Job drawing, mm, ordinate dimensions from the low corner. One solid piece. A direction names the side the tool comes from. Give positions to 0.01 mm unless a question says otherwise; leave off trailing zeros. Order: outer loops, then holes, each group sorted by start corner. A loop starts at its lowest first (then second) coordinate and runs counter-clockwise, first axis right, second up. Notation, with made-up numbers: M 58,40.25 L 70,40.25 A19 ccw 70,53.25 Z; hole C -1.75,-13 d11. An arc over 180 degrees is marked long. Put each result on its own line as item: value. Start each with the question number.
1) Cut at C-C (z = 23.5). Write the cut outline in (x, y), and give its area (3 significant figures).
2) Cut at A-A (y = 73). Write the cut outline in (x, z), and give its area (3 significant figures).
3) Two-plate mould, pull along Z, no slides. Class the marked faces 1, 2 and 3: released by +Z, released by -Z, zero draft, split by the parting line, or undercut.
4) Cut at D-D (x = 21.5). Write the cut outline in (y, z).
5) Cut at B-B (z = 33.5). Write the cut outline in (x, y), and give its area (3 significant figures).
6) Drill centre lines: line 1 (X direction, y = 73, z = 36.75); line 2 (Y direction, x = 15, z = 25.25); line 3 (Z direction, x = 2.25, y = 83.5). Where is each one in solid material? Low to high. Write a range as [from, to].
7) Pin check, flat tips, straight feed: pin 1 (3 mm diameter, centred on x = 15, y = 5, fed in from +Z); pin 2 (1.2 mm diameter, centred on x = 1.5, z = 29, fed in from +Y); pin 3 (1 mm diameter, centred on x = 26, z = 16, fed in from -Y); pin 4 (3 mm diameter, centred on x = 6, z = 26.5, fed in from -Y). Stop position of each tip, or through.
8) Tool access for the marked faces 4, 5 and 6: list every direction of +Z, -Z, +X, -X, +Y, -Y with a clear straight run to the whole face (end or side of a thin tool).
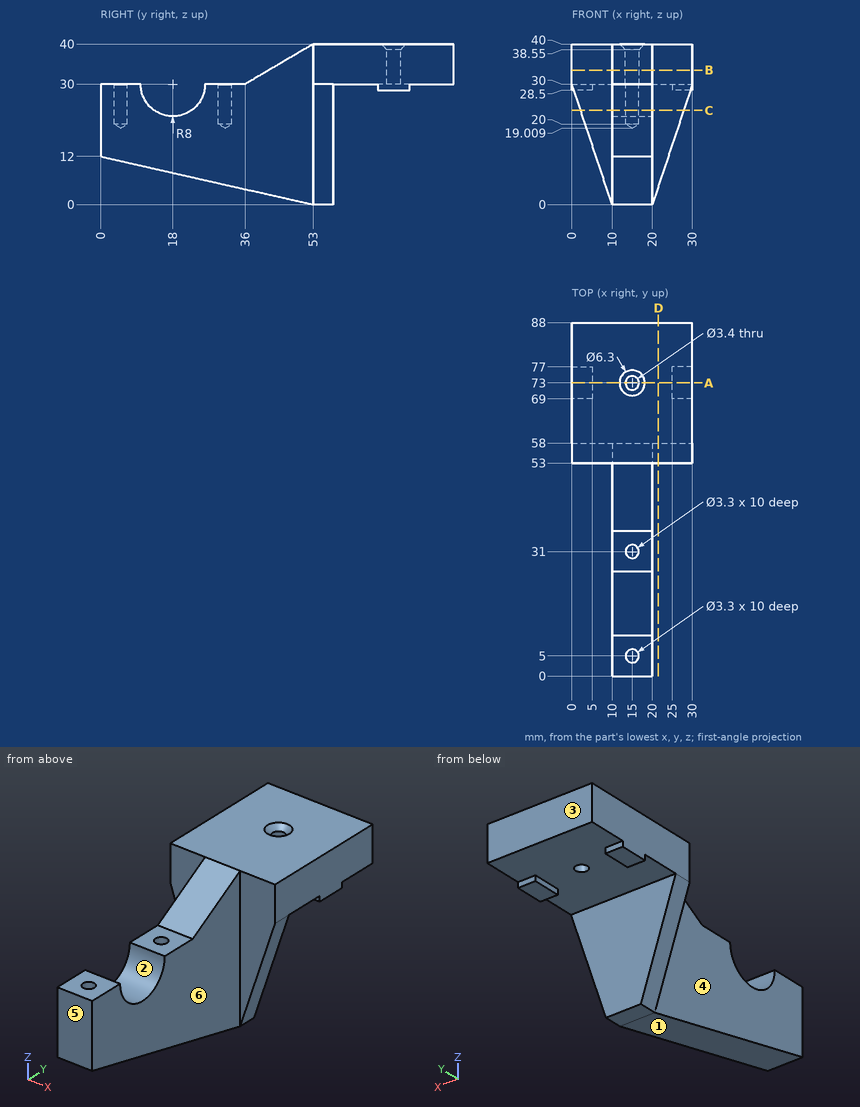
Solution:
1. outline: M 2.17,53 L 10,53 L 10,22.66 L 20,22.66 L 20,53 L 27.83,53 L 27.83,58 L 2.17,58 Z; M 10,0 L 20,0 L 20,13.34 L 10,13.34 Z; hole C 15,5 d3.3; hole C 15,31 d3.3
1. area: 548 mm²
2. outline: M 0,28.5 L 5,28.5 L 5,30 L 13.3,30 L 13.3,38.55 L 11.85,40 L 0,40 Z; M 16.7,30 L 25,30 L 25,28.5 L 30,28.5 L 30,40 L 18.15,40 L 16.7,38.55 Z
2. area: 279 mm²
3. face 1: released by -Z
3. face 2: released by +Z
3. face 3: zero draft
4. outline: M 53,4.5 L 58,4.5 L 58,30 L 88,30 L 88,40 L 53,40 Z
5. outline: M 0,53 L 10,53 L 10,41.95 L 20,41.95 L 20,53 L 30,53 L 30,88 L 0,88 Z; hole C 15,73 d3.4
5. area: 1,150 mm²
6. line 1: [0, 13.3], [16.7, 30]
6. line 2: [0, 3.35], [6.65, 11.56], [24.44, 29.35], [32.65, 58]
6. line 3: [30, 40]
7. pin 1: z = 19.91
7. pin 2: y = 77
7. pin 3: through
7. pin 4: y = 53
8. face 4: +Z, -Z, -X, -Y
8. face 5: +Z, -Z, +X, -X, -Y
8. face 6: +Z, -Z, +X, -Y
